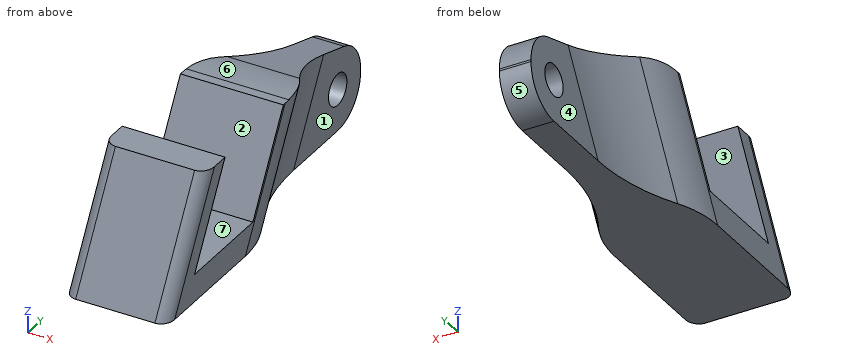
from build123d import *

# Parameters (mm, degrees)
F1_DEPTH     = 15
F3_DEPTH     = 25
F4_DEPTH     = 4.5
F6_DEPTH     = 4.5
F7_T4_DEPTH  = 80.5166313745
F7_T10_DEPTH = 80.5166313745
F8_SIZE2     = 20.5
F8_SIZE      = 6
F9_R         = 1.5
F10_R        = 10
F11_R        = 20
F12_R        = 5
F13_R        = 2
F14_DEPTH    = 25


# Not quite as in the source:
# - a fillet or chamfer that OpenCascade refuses, or shapes differently, is made with other operations: its cross-section is extruded or revolved along the edge and cut away or added


with BuildPart() as f1:
    # F0 (on Top) → F1 (new body)
    with BuildSketch(Plane.XY):
        Polygon((-6.5, 12), (-6.5, -25), (6.5, -25), (6.5, 12), (2, 12), (2, 25), (-2, 25), (-2, 12), align=None)
    extrude(amount=F1_DEPTH)

    # F2 (on face) → F3 (cut)
    with BuildSketch(Plane(origin=(-6.5, 0, 0), x_dir=(0, -1, 0), z_dir=(-1, 0, 0))):
        Polygon((6.2361162513, 3.5), (18.9378221735, 3.5), (12.2982940778, 15), (-0.4034118443, 15), align=None)
        Polygon((25, 15), (16.3397459622, 15), (25, 0), align=None)
    extrude(amount=-F3_DEPTH, mode=Mode.SUBTRACT)

    # F2 (on face) → F4 (cut)
    with BuildSketch(Plane(origin=(-6.5, 0, 0), x_dir=(0, -1, 0), z_dir=(-1, 0, 0))):
        Polygon((4.2153903092, 0), (2.194664367, 3.5), (-4.4448637287, 15), (-12, 15), (-12, 0), align=None)
    extrude(amount=-F4_DEPTH, mode=Mode.SUBTRACT)

    # F5 (on face) → F6 (cut)
    with BuildSketch(Plane.YZ.offset(6.5)):
        Polygon((12, 15), (4.4448637287, 15), (-4.2153903092, 0), (12, 0), align=None)
    extrude(amount=-F6_DEPTH, mode=Mode.SUBTRACT)

    # F7: fillet of radius 20 on 2 edges, made by hand


with BuildPart() as f7_tool2:
    # F7_s3 → F7_t4 (new body)
    with BuildSketch(Plane(origin=(0, -16.852878402, -29.190041646), x_dir=(1, 0, 0), z_dir=(0, 0.5, 0.8660254038))):
        with BuildLine():
            ThreePointArc((-6.5, -3.6506350946), (-3.1585563186, 2.2803856327), (-2, 8.9885895652))
            Line((-2, 8.9885895652), (-2, -3.6506350946))
            Line((-2, -3.6506350946), (-6.5, -3.6506350946))
        make_face()
    extrude(amount=F7_T4_DEPTH)

    split(bisect_by=Plane.XY.offset(15), keep=Keep.BOTTOM)

    split(bisect_by=Plane.XY, keep=Keep.TOP)


with BuildPart() as f1_1:
    add(f1.part)

    # F7_t1: union F7_tool2
    add(f7_tool2.part)


with BuildPart() as f7_tool8:
    # F7_s9 → F7_t10 (new body)
    with BuildSketch(Plane(origin=(0, 23.4054372853, 40.5394065514), x_dir=(1, 0, 0), z_dir=(0, -0.5, -0.8660254038))):
        with BuildLine():
            ThreePointArc((6.5, 3.6506350946), (3.1585563186, -2.2803856327), (2, -8.9885895652))
            Line((2, -8.9885895652), (2, 3.6506350946))
            Line((2, 3.6506350946), (6.5, 3.6506350946))
        make_face()
    extrude(amount=F7_T10_DEPTH)

    split(bisect_by=Plane.XY, keep=Keep.TOP)

    split(bisect_by=Plane.XY.offset(15), keep=Keep.BOTTOM)


with BuildPart() as f1_2:
    add(f1_1.part)

    # F7_t7: union F7_tool8
    add(f7_tool8.part)

    # F8
    f8_edges = [f1_2.edges().sort_by_distance(p)[0] for p in [
        (0, 25, 15),
    ]]
    f8_side = f1_2.faces().sort_by_distance((0, 25, 7.5))[0]
    chamfer(f8_edges, length=F8_SIZE, length2=F8_SIZE2, reference=f8_side)

    # F9
    f9_edges = [f1_2.edges().sort_by_distance(p)[0] for p in [
        (-6.5, -20.669873, 7.5),
        (6.5, -20.669873, 7.5),
    ]]
    fillet(f9_edges, radius=F9_R)

    # F10
    f10_edges = [f1_2.edges().sort_by_distance(p)[0] for p in [
        (-6.5, 0.114737, 7.5),
        (6.5, 0.114737, 7.5),
    ]]
    fillet(f10_edges, radius=F10_R)

    # F11
    f11_edges = [f1_2.edges().sort_by_distance(p)[0] for p in [
        (0, 4.5, 15),
    ]]
    fillet(f11_edges, radius=F11_R)

    # F12
    f12_edges = [f1_2.edges().sort_by_distance(p)[0] for p in [
        (0, 25, 9),
        (0, 25, 0),
    ]]
    fillet(f12_edges, radius=F12_R)

    # F13 (on face) → F14 (cut)
    with BuildSketch(Plane.YZ.offset(2)):
        with Locations((20, 5.2536562529)):
            Circle(F13_R)
    extrude(amount=-F14_DEPTH, mode=Mode.SUBTRACT)


solid = f1_2.part
Could you check a few things on this model? Use its own coordinates, in mm. Face numbers are marked on the shaded views. A direction names the side the tool comes from. Give positions to 0.01 mm unless a question says otherwise; leave off trailing zeros. Write each loop counter-clockwise with the first axis right and the second up, starting at its lowest first coordinate (ties: lowest second). Pieces come first, ordered by that corner, then holes. Notation, with made-up numbers: (72.5, 44.25) -> (82.5, 44.25) arc R21 ccw to (82.5, 69.25) -> close; hole circle Ø1 at (65.5, -5). An arc over 180 degrees is marked (long way). Write each question's results on one line, items separated by ' | '. Start each with the question number.
Q1. Which directions (+Z, -Z, +X, -X, +Y, -Y) give clear straight access to the entire face, cutting with the end or side of a thin tool? Please do the marked faces 1, 2, 3 and 4.
Q2. Suppose I cut it at A-A, the plane x = -0.5. List the corners of the cut face in (y, z) for me.
Q3. We'd pull the mould along Z, two halves only. Please class the marked faces 5, 6 and 7: +Z half, -Z half, draft (parallel to the pull), parting line (faces both ways), or undercut.
Q4. Suppose I cut it at B-B, the plane y = 19. List the corners of the cut face in (x, z) for me, and give its area (3 significant figures).
Q5. Suppose I cut it at C-C, the plane x = -4. List the corners of the cut face in (y, z) for me, and give its area (3 significant figures).
Q6. I need wall thicknesses on probe 1 along Y at (x, z) = (5, 12.5); probe 2 along Z at (x, y) = (-0.15, 20); probe 3 along Y at (x, z) = (0.75, 5.25). Which ranges of each line are inside material? Lowest first, please.
Q7. I'm going to push flat-ended pins straight in: pin 1 Ø8 at (y, z) = (18, 6.5) entering from +X; pin 2 Ø2 at (x, z) = (-2.5, 9.5) entering from -Y; pin 3 Ø2 at (x, z) = (3.5, 11.5) entering from -Y. Where does each tip first touch, or does it pass through?
Outcome:
1) face 1: -Z, +X, +Y | face 2: +Z, +X, -X | face 3: +X, -X | face 4: -Z, -X, +Y
2) outline: (-25, 0) -> (20, 0) arc R5 ccw to (25, 5) -> (25, 5.25) arc R5 ccw to (21.4, 10.05) -> (7.25, 14.19) arc R20 ccw to (1.63, 15) -> (0.4, 15) -> (-6.24, 3.5) -> (-18.94, 3.5) -> (-12.3, 15) -> (-16.34, 15) -> close; hole circle Ø4 at (20, 5.25)
3) face 5: -Z half | face 6: +Z half | face 7: undercut
4) outline: (-2, 0) -> (2, 0) -> (2, 3.52) -> (-2, 3.52) -> close; (-2, 6.99) -> (2, 6.99) -> (2, 10.76) -> (-2, 10.76) -> close | area: 29.2 mm2
5) outline: (-25, 0) -> (0.31, 0) -> (8.33, 13.88) -> (7.25, 14.19) arc R20 ccw to (1.63, 15) -> (0.4, 15) -> (-6.24, 3.5) -> (-18.94, 3.5) -> (-12.3, 15) -> (-16.34, 15) -> close | area: 231 mm2
6) probe 1: -17.78 to -13.74, -1.04 to 5.43 | probe 2: 0 to 3.25, 7.25 to 10.46 | probe 3: -21.97 to -17.93, -5.23 to 18, 22 to 25
7) pin 1: x = 2.01 | pin 2: y = -20.09 | pin 3: y = -18.94
